from build123d import *

# Parameters (mm, degrees)
BOSS_EXTRUDE1_DEPTH = 40
CUT_EXTRUDE1_START  = -20
CUT_EXTRUDE1_DEPTH  = 20
CUT_EXTRUDE2_REACH  = 114.942
SKETCH3_R           = 4


with BuildPart() as part:
    # Sketch1 → Boss-Extrude1 (new body)
    with BuildSketch(Plane.XY):
        with BuildLine():
            Line((0, 6), (0, 0))
            Line((0, 0), (29, 0))
            ThreePointArc((29, 0), (33.242640687, 1.757359313), (35, 6))
            Line((35, 6), (35, 31))
            ThreePointArc((35, 31), (35.878679656, 33.121320344), (38, 34))
            Line((38, 34), (62, 34))
            ThreePointArc((62, 34), (64.121320344, 33.121320344), (65, 31))
            Line((65, 31), (65, 6))
            ThreePointArc((65, 6), (66.757359313, 1.757359313), (71, 0))
            Line((71, 0), (100, 0))
            Line((100, 0), (100, 6))
            Line((100, 6), (74, 6))
            ThreePointArc((74, 6), (71.878679656, 6.878679656), (71, 9))
            Line((71, 9), (71, 34))
            ThreePointArc((71, 34), (69.242640687, 38.242640687), (65, 40))
            Line((65, 40), (35, 40))
            ThreePointArc((35, 40), (30.757359313, 38.242640687), (29, 34))
            Line((29, 34), (29, 9))
            ThreePointArc((29, 9), (28.121320344, 6.878679656), (26, 6))
            Line((26, 6), (0, 6))
        make_face()
    extrude(amount=BOSS_EXTRUDE1_DEPTH)

    # Sketch2 → Cut-Extrude1 (cut)
    with BuildSketch(Plane.XY.offset(40).offset(CUT_EXTRUDE1_START)):
        with BuildLine():
            Line((29, 20), (35, 20))
            Line((35, 20), (35, 31))
            ThreePointArc((35, 31), (35.878679656, 33.121320344), (38, 34))
            Line((38, 34), (62, 34))
            ThreePointArc((62, 34), (64.121320344, 33.121320344), (65, 31))
            Line((65, 31), (65, 20))
            Line((65, 20), (71, 20))
            Line((71, 20), (71, 34))
            ThreePointArc((71, 34), (69.242640687, 38.242640687), (65, 40))
            Line((65, 40), (35, 40))
            ThreePointArc((35, 40), (30.757359313, 38.242640687), (29, 34))
            Line((29, 34), (29, 20))
        make_face()
    extrude(amount=CUT_EXTRUDE1_DEPTH, mode=Mode.SUBTRACT)

    # Sketch3 → Cut-Extrude2 (cut, up to next)
    with BuildSketch(Plane(origin=(0, 6, 0), x_dir=(1, 0, 0), z_dir=(0, 1, 0)), mode=Mode.PRIVATE) as cut_extrude2_sk1:
        with Locations(Location((12, -12, 0), (0, 0, 180))):
            Circle(SKETCH3_R)
    cut_extrude2_tool1 = extrude(cut_extrude2_sk1.sketch, amount=-CUT_EXTRUDE2_REACH, mode=Mode.PRIVATE) & part.part
    # Sketch3 → Cut-Extrude2 (cut, up to next)
    with BuildSketch(Plane(origin=(0, 6, 0), x_dir=(1, 0, 0), z_dir=(0, 1, 0)), mode=Mode.PRIVATE) as cut_extrude2_sk2:
        with Locations(Location((12, -28, 0), (0, 0, 180))):
            Circle(SKETCH3_R)
    cut_extrude2_tool2 = extrude(cut_extrude2_sk2.sketch, amount=-CUT_EXTRUDE2_REACH, mode=Mode.PRIVATE) & part.part
    # Sketch3 → Cut-Extrude2 (cut, up to next)
    with BuildSketch(Plane(origin=(0, 6, 0), x_dir=(1, 0, 0), z_dir=(0, 1, 0)), mode=Mode.PRIVATE) as cut_extrude2_sk3:
        with Locations(Location((88, -12, 0), (0, 0, 180))):
            Circle(SKETCH3_R)
    cut_extrude2_tool3 = extrude(cut_extrude2_sk3.sketch, amount=-CUT_EXTRUDE2_REACH, mode=Mode.PRIVATE) & part.part
    # Sketch3 → Cut-Extrude2 (cut, up to next)
    with BuildSketch(Plane(origin=(0, 6, 0), x_dir=(1, 0, 0), z_dir=(0, 1, 0)), mode=Mode.PRIVATE) as cut_extrude2_sk4:
        with Locations(Location((88, -28, 0), (0, 0, 180))):
            Circle(SKETCH3_R)
    cut_extrude2_tool4 = extrude(cut_extrude2_sk4.sketch, amount=-CUT_EXTRUDE2_REACH, mode=Mode.PRIVATE) & part.part
    add(cut_extrude2_tool1.solids().sort_by_distance((12, 6, 12))[0], mode=Mode.SUBTRACT)
    add(cut_extrude2_tool2.solids().sort_by_distance((12, 6, 28))[0], mode=Mode.SUBTRACT)
    add(cut_extrude2_tool3.solids().sort_by_distance((88, 6, 12))[0], mode=Mode.SUBTRACT)
    add(cut_extrude2_tool4.solids().sort_by_distance((88, 6, 28))[0], mode=Mode.SUBTRACT)


solid = part.part
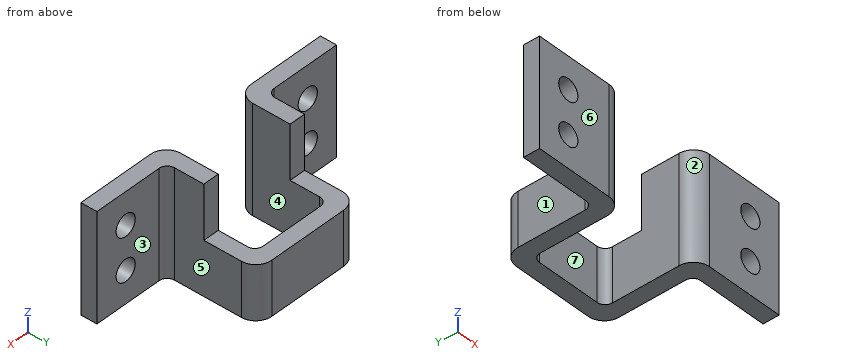
Check sheet for the modelled part. Datum: model origin and axes. Units: mm. Face numbers are marked on the shaded views. A direction names the side the tool comes from. Round coordinates to 2 decimals unless told otherwise and drop trailing zeros. Write each loop counter-clockwise with the first axis right and the second up, starting at its lowest first coordinate (ties: lowest second). Pieces come first, ordered by that corner, then holes. Notation, with made-up numbers: (-5.5, 28.5) - (16.5, 28.5) arc R18 ccw to (16.5, 50.5) - close; hole circle Ø11 at (19.5, 34). An arc over 180 degrees is marked (long way). Return JSON: item names as keys, results as strings.
Q1. Access from +Z, -Z, +X, -X, +Y, -Y to the whole of each face (thin tool, end or side, straight path). Record for the marked faces 1, 2 and 3.
Returned:
{"face 1": "+Z, -Z, -X, +Y", "face 2": "+Z, -Z, -Y", "face 3": "+Z, -Z, +X, +Y"}
Q2. Cross-section at C-C (y = 16.5). Record the boundary of the cut face in (x, z), then the cut area to 3 significant figures.
Returned:
{"outline": "(29, 0) - (35, 0) - (35, 40) - (29, 40) - close; (65, 0) - (71, 0) - (71, 40) - (65, 40) - close", "area": "480 mm²"}
Q3. Draft check along X on the marked faces 4, 5, 6 and 7. Enter one of: released by +X, released by -X, zero draft, split by the parting line, or undercut.
Returned:
{"face 4": "undercut", "face 5": "released by +X", "face 6": "zero draft", "face 7": "undercut"}
Q4. Cross-section at A-A (x = 12). Record the boundary of the cut face in (y, z).
Returned:
{"outline": "(0, 0) - (6, 0) - (6, 8) - (0, 8) - close; (0, 16) - (6, 16) - (6, 24) - (0, 24) - close; (0, 32) - (6, 32) - (6, 40) - (0, 40) - close"}
Q5. Cross-section at D-D (z = 28). Record the boundary of the cut face in (x, y).
Returned:
{"outline": "(0, 0) - (8, 0) - (8, 6) - (0, 6) - close; (16, 0) - (29, 0) arc R6 ccw to (35, 6) - (35, 20) - (29, 20) - (29, 9) arc R3 cw to (26, 6) - (16, 6) - close; (65, 6) arc R6 ccw to (71, 0) - (84, 0) - (84, 6) - (74, 6) arc R3 cw to (71, 9) - (71, 20) - (65, 20) - close; (92, 0) - (100, 0) - (100, 6) - (92, 6) - close"}
Q6. Scan lines: L1, parallel to Z at x = 12, y = 2; L2, parallel to X at y = 16, z = 33; L3, parallel to Y at x = 52, z = 15.5. Record each from-to range of solid material in increasing order. Write a range as from..to.
Returned:
{"L1": "z = 0..8, 16..24, 32..40", "L2": "x = 29..35, 65..71", "L3": "y = 34..40"}
Q7. Cross-section at B-B (z = 36). Record the boundary of the cut face in (x, y).
Returned:
{"outline": "(0, 0) - (29, 0) arc R6 ccw to (35, 6) - (35, 20) - (29, 20) - (29, 9) arc R3 cw to (26, 6) - (0, 6) - close; (65, 6) arc R6 ccw to (71, 0) - (100, 0) - (100, 6) - (74, 6) arc R3 cw to (71, 9) - (71, 20) - (65, 20) - close"}
Q8. Depth check by flat-ended pin: P1, Ø13, axis at x = 12, z = 12, coming from the -Y side; P2, Ø6.5, axis at x = 66.5, z = 31.5, coming from the +Y side; P3, Ø8, axis at x = 13, z = 24, coming from the +Y side; P4, Ø6.5, axis at x = 12, z = 28, coming from the -Y side. Enter the tip coordinate at first touch or a pass-through.
Returned:
{"P1": "stops at y = 0", "P2": "stops at y = 20", "P3": "stops at y = 6", "P4": "passes through"}
